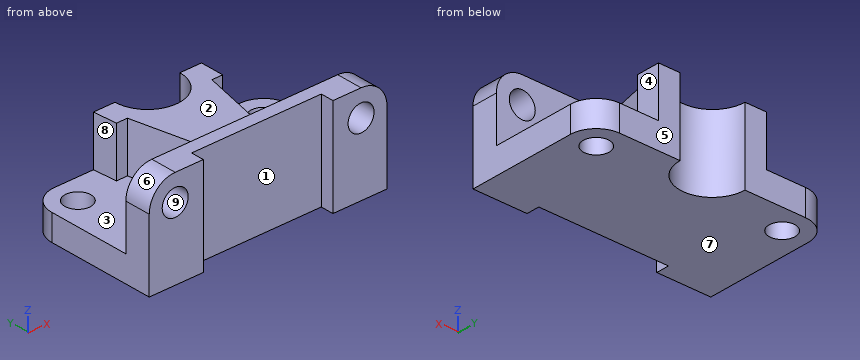
```python
from build123d import *

# Parameters (mm, degrees)
BOSS_EXTRUDE1_DEPTH = 110
BOSS_EXTRUDE2_DEPTH = 23
CUT_EXTRUDE1_START  = -23
CUT_EXTRUDE1_DEPTH  = 23
SKETCH6_W           = 60
SKETCH6_H           = 6
CUT_EXTRUDE2_DEPTH  = 153
FILLET1_R           = 12
SKETCH9_R           = 6
CUT_EXTRUDE3_DEPTH  = 153
FILLET3_R           = 12
SKETCH10_R          = 6
CUT_EXTRUDE4_DEPTH  = 153
SKETCH11_R          = 6
CUT_EXTRUDE5_DEPTH  = 153


with BuildPart() as part:
    # Sketch1 → Boss-Extrude1 (new body)
    with BuildSketch(Plane(origin=(0, 0, 0), x_dir=(0, 0, -1), z_dir=(1, 0, 0))):
        Polygon((0, 0), (0, -62), (-45, -62), (-45, -50), (-12, -50), (-12, 0), align=None)
    extrude(amount=BOSS_EXTRUDE1_DEPTH)

    # Sketch4 → Boss-Extrude2 (add)
    with BuildSketch(Plane.XY.offset(12)):
        with BuildLine():
            Line((30, 0), (40, 0))
            ThreePointArc((40, 0), (55, -15), (70, 0))
            Line((70, 0), (80, 0))
            Line((80, 0), (80, -10.913379379))
            Line((80, -10.913379379), (75, -10.913379379))
            Line((75, -10.913379379), (66, -50))
            Line((66, -50), (44, -50))
            Line((44, -50), (35.902837649, -10.913379379))
            Line((35.902837649, -10.913379379), (30.855515073, -10.913379379))
            Line((30.855515073, -10.913379379), (30, 0))
        make_face()
    extrude(amount=BOSS_EXTRUDE2_DEPTH)

    # Sketch5 → Cut-Extrude1 (cut)
    with BuildSketch(Plane.XY.offset(12).offset(CUT_EXTRUDE1_START)):
        with BuildLine():
            Line((70, 0), (40, 0))
            ThreePointArc((40, 0), (55, -15), (70, 0))
        make_face()
    extrude(amount=CUT_EXTRUDE1_DEPTH, mode=Mode.SUBTRACT)

    # Sketch6 → Cut-Extrude2 (cut)
    with BuildSketch(Plane.XY.offset(45)):
        with Locations((55, -59)):
            Rectangle(SKETCH6_W, SKETCH6_H)
    extrude(amount=-CUT_EXTRUDE2_DEPTH, mode=Mode.SUBTRACT)

    # Fillet1
    fillet1_edges = [part.edges().sort_by_distance(p)[0] for p in [
        (110, -56, 45),
        (0, -56, 45),
    ]]
    fillet(fillet1_edges, radius=FILLET1_R)

    # Sketch9 → Cut-Extrude3 (cut)
    with BuildSketch(Plane(origin=(0, -50, 0), x_dir=(1, 0, 0), z_dir=(0, 1, 0))):
        with Locations(Location((12, -33, 0), (0, 0, 270))):
            Circle(SKETCH9_R)
    cut_extrude3 = extrude(amount=-CUT_EXTRUDE3_DEPTH, mode=Mode.SUBTRACT)

    # Mirror1: Cut-Extrude3 across plane
    add(cut_extrude3.mirror(Plane.ZY.offset(-55)), mode=Mode.SUBTRACT)

    # Fillet3
    fillet3_edges = [part.edges().sort_by_distance(p)[0] for p in [
        (110, 0, 6),
        (0, 0, 6),
    ]]
    fillet(fillet3_edges, radius=FILLET3_R)

    # Sketch10 → Cut-Extrude4 (cut)
    with BuildSketch(Plane(origin=(0, 0, 0), x_dir=(-1, 0, 0), z_dir=(0, 0, -1))):
        with Locations((-12, -12)):
            Circle(SKETCH10_R)
    extrude(amount=-CUT_EXTRUDE4_DEPTH, mode=Mode.SUBTRACT)

    # Sketch11 → Cut-Extrude5 (cut)
    with BuildSketch(Plane.XY.offset(12)):
        with Locations((98, -12)):
            Circle(SKETCH11_R)
    extrude(amount=-CUT_EXTRUDE5_DEPTH, mode=Mode.SUBTRACT)


solid = part.part
```
Geometry check sheet. Reference: the model listing, model coordinates, mm. Face numbers are marked on the shaded views. A direction names the side the tool comes from. Round coordinates to 2 decimals unless told otherwise and drop trailing zeros. Order: outer loops, then holes, each group sorted by start corner. A loop starts at its lowest first (then second) coordinate and runs counter-clockwise, first axis right, second up. Notation, with made-up numbers: (-26.5, 62) - (6.5, 62) arc R16 ccw to (6.5, 69) - close; hole circle Ø7 at (-21.5, -0.5). An arc over 180 degrees is marked (long way). Use a Markdown table: item, result. Add a question column.
1) Gauge pin test, flat ends, axial feed: P1, Ø8, axis at y = -14.5, z = 12.5, coming from the -X side; P2, Ø19, axis at x = 12, y = -12, coming from the +Z side; P3, Ø6, axis at x = 36, y = -17, coming from the +Z side; P4, Ø1.5, axis at x = 77.5, z = 23.5, coming from the -Y side. Record the tip position at first contact, or that the pin passes through.
2) Section check D-D (x = 27.5). Record the cut outline in (y, z).
3) Thickness scan on line 1 along X through (y, z) = (-54, 33); line 2 along X through (y, z) = (-58.5, 33); line 3 along Y through (x, z) = (12, 9). Record the ranges inside material, lowest first.
4) Set-up check for the marked faces 1, 2, 3, 4 and 5: record each of +Z, -Z, +X, -X, +Y, -Y from which the full face is reachable in a straight line by a thin tool's end or side.
5) Section check C-C (z = 31). Record the cut outline in (x, y).
6) Section check A-A (z = 10). Record the cut outline in (x, y), then the cut area to 3 significant figures.
7) Mould release check, pull along Z, two halves, no side actions. Record for the marked faces 6, 7, 8 and 9: released by +Z, released by -Z, zero draft, split by the parting line, or undercut.
8) Section check B-B (y = -7.5). Record the cut outline in (x, z), then the cut area to 3 significant figures.
Established:
| question | item | result |
|---|---|---|
| 1 | P1 | x = 0 |
| 1 | P2 | z = 12 |
| 1 | P3 | z = 35 |
| 1 | P4 | y = -56 |
| 2 | outline | (-56, 0) - (0, 0) - (0, 12) - (-50, 12) - (-50, 45) - (-56, 45) - close |
| 3 | line 1 | 0 to 6, 18 to 92, 104 to 110 |
| 3 | line 2 | 0 to 6, 18 to 25, 85 to 92, 104 to 110 |
| 3 | line 3 | -62 to -18, -6 to 0 |
| 4 | face 1 | +Z, -Z, -Y |
| 4 | face 2 | +Z, +X, -X, +Y |
| 4 | face 3 | +Z, -X |
| 4 | face 4 | +Z, +X, +Y |
| 4 | face 5 | +Z, -Z, +X, -X, +Y |
| 5 | outline | (0, -62) - (6.34, -62) - (6.34, -50) - (0, -50) - close; (17.66, -62) - (25, -62) - (25, -56) - (85, -56) - (85, -62) - (92.34, -62) - (92.34, -50) - (66, -50) - (75, -10.91) - (80, -10.91) - (80, 0) - (70, 0) arc R15 cw to (40, 0) - (30, 0) - (30.86, -10.91) - (35.9, -10.91) - (44, -50) - (17.66, -50) - close; (103.66, -62) - (110, -62) - (110, -50) - (103.66, -50) - close |
| 6 | outline | (0, -62) - (25, -62) - (25, -56) - (85, -56) - (85, -62) - (110, -62) - (110, -12) arc R12 ccw to (98, 0) - (70, 0) arc R15 cw to (40, 0) - (12, 0) arc R12 ccw to (0, -12) - close; hole circle Ø12 at (12, -12); hole circle Ø12 at (98, -12) |
| 6 | area | 5,820 mm2 |
| 7 | face 6 | released by +Z |
| 7 | face 7 | released by -Z |
| 7 | face 8 | zero draft |
| 7 | face 9 | undercut |
| 8 | outline | (0.88, 0) - (8.03, 0) - (8.03, 12) - (0.88, 12) - close; (15.97, 0) - (42.01, 0) - (42.01, 35) - (30.59, 35) - (30.59, 12) - (15.97, 12) - close; (67.99, 0) - (94.03, 0) - (94.03, 12) - (80, 12) - (80, 35) - (67.99, 35) - close; (101.97, 0) - (109.12, 0) - (109.12, 12) - (101.97, 12) - close |
| 8 | area | 1,340 mm2 |
